Design review of the part built by this model. Coordinates are the model's own, in mm. Face numbers are marked on the shaded views. A direction names the side the tool comes from. Give positions to 0.01 mm unless a question says otherwise; leave off trailing zeros. Loops run counter-clockwise (first coordinate to the right, second up) from the corner with the lowest first, then second, coordinate; pieces in that order, holes last. Notation, with made-up numbers: (55, 32) - (102, 32) arc R12 cw to (102, 40) - close; hole circle Ø3 at (-32.75, -32.5). An arc over 180 degrees is marked (long way). Write each question's results on one line, items separated by ' | '.
Autodesk Inventor part; units mm, degrees
ref_plane "YZ Plane" through (0, 0, 0) normal (1, 0, 0) x (0, 1, 0)
ref_plane "XZ Plane" through (0, 0, 0) normal (0, 1, 0) x (-1, 0, 0)
ref_plane "XY Plane" through (0, 0, 0) normal (0, 0, 1) x (1, 0, 0)
sketch "Sketch1" plane through (0, 0, 0) normal (1, 0, 0) x (0, 1, 0)
  circle A0 centre (0, 0) radius 11
  circle A1 centre (0, 0) radius 8.5
  line L0 (2.5, 10.712143) -> (-2.5, 10.712143)
  line L1 (-2.5, 10.712143) -> (-2.5, -10.712143)
  line L2 (-2.5, -10.712143) -> (2.5, -10.712143)
  line L3 (2.5, -10.712143) -> (2.5, 10.712143)
  line L4 (2.5, 10.712143) -> (-2.5, -10.712143) construction
  line L5 (-2.5, 10.712143) -> (2.5, -10.712143) construction
  dimension "d0" = 22
  dimension "d3" = 17
  dimension "d18" = 5
extrude "Extrusion1" add sketch "Sketch1" along normal blind 12 contours A0 L3 A1 | L3 A1 L1 L0 | L2 L1 A1 L3 | L1 A1 A0
sketch "Sketch2" plane through (0, 0, 0) normal (0, 0, 1) x (1, 0, 0)
  line L0 (14.5, 2.5) -> (9.5, 2.5)
  line L1 (9.5, 2.5) -> (9.5, -2.5)
  line L2 (9.5, -2.5) -> (14.5, -2.5)
  line L3 (14.5, -2.5) -> (14.5, 2.5)
  line L4 (14.5, 2.5) -> (9.5, -2.5) construction
  line L5 (9.5, 2.5) -> (14.5, -2.5) construction
  circle A0 centre (9.5, 0) radius 2.5
  line L6 (12, -2.5) -> (12, 2.5)
  point P0 (0, 0)
  point P1 (9.5, 2.5)
  point P2 (12, 0)
  dimension "d4" = 5
  dimension "d5" = 5
extrude "Extrusion2" add sketch "Sketch2" along normal mid plane 34 contours L6 A0 L0 | A0 L1 | L1 A0 | L6 L2 A0
sketch "Sketch3" plane through (12, 0, 0) normal (1, 0, 0) x (0, 0, -1)
  circle A0 centre (0, 0) radius 9.5
  dimension "d8" = 19
extrude "Extrusion3" cut sketch "Sketch3" against normal blind 10.5
chamfer "Chamfer1" distance 1 angle 45 4 edges at (0, -11, 0) (0, 11, 0) (0, 0, -10.7121) (0, 0, 10.7121)
sketch "Sketch4" plane through (0, 0, 0) normal (0, 1, 0) x (-1, 0, 0)
  line L0 (-12, 10.712143) -> (-12, -10.712143)
  circle A0 centre (-24, 0) radius 16.085708
  line L1 (-12, 0) -> (-24, 0) construction
  point P0 (0, 0)
  point P1 (-12, 10.712143)
  dimension "d14" = 12
extrude "Extrusion4" cut sketch "Sketch4" along normal through all both and the other way through all contours A0 L0 picked at (-11.258553, -2.503733)
fillet "Fillet1" radius 2 2 edges at (12, 0, -10.7121) (12, 0, 10.7121)
properties part number "Cup" material "Aluminum 6061"
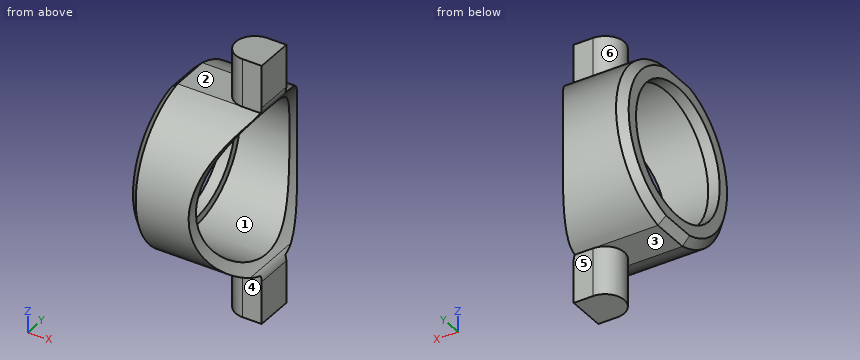
(1) Take a section at A-A on z = 0. Give the boundary of the cut face in (x, y), plus the area to 3 significant figures.
Answers below:
outline: (0, -10) - (1, -11) - (7.91, -11) - (7.91, -9.5) - (1.5, -9.5) - (1.5, -8.5) - (0, -8.5) - close; (0, 8.5) - (1.5, 8.5) - (1.5, 9.5) - (7.91, 9.5) - (7.91, 11) - (1, 11) - (0, 10) - close | area: 25.7 mm2
(2) Take a section at C-C on x = 5.5. Give the boundary of the cut face in (y, z).
Answers below:
outline: (-2.5, -10.71) - (2.5, -10.71) arc R11 ccw to (2.5, 10.71) - (-2.5, 10.71) arc R11 ccw to start; hole circle Ø19 at (0, 0)
(3) Draft analysis for pull direction Z (two halves, no side actions). For the marked faces 1, 2 and 3, state which applies: pulls with the +Z half, pulls with the -Z half, needs draft (parallel to the pull), parting line crosses it, or undercut.
Answers below:
face 1: undercut | face 2: pulls with the +Z half | face 3: pulls with the -Z half
(4) Wall thickness on line 1 along Z through (x, y) = (4, 0); line 2 along Y through (x, z) = (1.2, 0); line 3 along Z through (x, y) = (0.95, 0): over which ranges is each line inside the solid? List them lowest first. Write a range as from..to.
Answers below:
line 1: -10.71..-9.5, 9.5..10.71 | line 2: -11..-8.5, 8.5..11 | line 3: -10.66..-8.5, 8.5..10.66
(5) Take a section at B-B on y = 0. Give the boundary of the cut face in (x, z), plus the area to 3 significant figures.
Answers below:
outline: (0, -9.71) - (1, -10.71) - (7, -10.71) - (7, -17) - (12, -17) - (12, -11.45) arc R2 ccw to (11.55, -10.18) arc R16.09 cw to (11.02, -9.5) - (1.5, -9.5) - (1.5, -8.5) - (0, -8.5) - close; (0, 8.5) - (1.5, 8.5) - (1.5, 9.5) - (11.02, 9.5) arc R16.09 cw to (11.55, 10.18) arc R2 ccw to (12, 11.45) - (12, 17) - (7, 17) - (7, 10.71) - (1, 10.71) - (0, 9.71) - close | area: 92.6 mm2
(6) Take a section at D-D on z = 14. Give the boundary of the cut face in (x, y).
Answers below:
outline: (9.5, -2.5) - (12, -2.5) - (12, 2.5) - (9.5, 2.5) arc R2.5 ccw to start
(7) Insertion check: P1, Ø0.8, axis at x = 10.5, z = 15, coming from the +Y side; P2, Ø1.5, axis at x = 7, y = -3.5, coming from the -Z side; P3, Ø0.8, axis at x = 11, z = -14.5, coming from the -Y side; P4, Ø1, axis at y = -3, z = -5.5, coming from the +X side. Each pin has a flat end and moves straight along its axis. Give the tip position at first contact, or say it passes through.
Answers below:
P1: y = 2.5 | P2: z = -10.65 | P3: y = -2.5 | P4: through
(8) Tool access review of the marked faces 4, 5 and 6: name each direction out of +Z, -Z, +X, -X, +Y, -Y from which nothing blocks a thin tool from reaching the whole face with its end or side.
Answers below:
face 4: -Z, +X, -X, -Y | face 5: -Z, +X, -X, +Y | face 6: +Z, -X
